```python
from build123d import *

# Parameters (mm, degrees)
BODY_MOVE_COPY1_START         = -65
BODY_MOVE_COPY1_OUTLINE_W     = 5.1
BODY_MOVE_COPY1_OUTLINE_H     = 30.1
BODY_MOVE_COPY1_OUTLINE_R     = 2.6
BODY_MOVE_COPY1_OUTLINE_R_2   = 3.1
BODY_MOVE_COPY1_OUTLINE_R_3   = 1.55
BODY_MOVE_COPY1_OUTLINE_W_2   = 30.5
BODY_MOVE_COPY1_OUTLINE_H_2   = 14.5
BODY_MOVE_COPY1_DEPTH         = 5
BODY_MOVE_COPY1_START_2       = -5
BODY_MOVE_COPY1_2_OUTLINE_W   = 10
BODY_MOVE_COPY1_2_OUTLINE_H   = 5.2
BODY_MOVE_COPY1_2_OUTLINE_R   = 1.6
BODY_MOVE_COPY1_2_OUTLINE_W_2 = 5.1
BODY_MOVE_COPY1_2_OUTLINE_H_2 = 30.1
BODY_MOVE_COPY1_2_DEPTH       = 5
SKETCH26_W                    = 10
SKETCH26_H                    = 5.2
BOSS_EXTRUDE2_DEPTH           = 5
SKETCH28_W                    = 5.1
SKETCH28_H                    = 30.1
CUT_EXTRUDE1_DEPTH            = 349.066085679


# Read off the part's stored shape, not the designer's step: Body-Move/Copy1
with BuildPart() as part:
    # Body-Move/Copy1 outline → Body-Move/Copy1 (new body)
    with BuildSketch(Plane.XY.offset(BODY_MOVE_COPY1_START)):
        Polygon((24.9, -310), (24.9, -305), (100.2, -305), (100.2, -310), (150, -310), (150, -5), (10.65, -5), (10.65, 0), (-10.65, 0), (-10.65, -5), (-150, -5), (-150, -310), (-100.2, -310), (-100.2, -305), (-24.9, -305), (-24.9, -310), align=None)
        with Locations((-143.45, -280)):
            Rectangle(BODY_MOVE_COPY1_OUTLINE_W, BODY_MOVE_COPY1_OUTLINE_H, mode=Mode.SUBTRACT)
        with Locations((-90, -157.5)):
            Circle(BODY_MOVE_COPY1_OUTLINE_R, mode=Mode.SUBTRACT)
        with Locations((-60, -157.5)):
            Circle(BODY_MOVE_COPY1_OUTLINE_R, mode=Mode.SUBTRACT)
        with Locations((143.45, -280)):
            Rectangle(BODY_MOVE_COPY1_OUTLINE_W, BODY_MOVE_COPY1_OUTLINE_H, mode=Mode.SUBTRACT)
        with Locations((65, -157.5)):
            Circle(BODY_MOVE_COPY1_OUTLINE_R_2, mode=Mode.SUBTRACT)
        with Locations((85, -157.5)):
            Circle(BODY_MOVE_COPY1_OUTLINE_R_2, mode=Mode.SUBTRACT)
        with Locations((-90, -137.5)):
            Circle(BODY_MOVE_COPY1_OUTLINE_R_3, mode=Mode.SUBTRACT)
        with Locations((-60, -137.5)):
            Circle(BODY_MOVE_COPY1_OUTLINE_R_3, mode=Mode.SUBTRACT)
        with Locations((-75, -100.25)):
            Rectangle(BODY_MOVE_COPY1_OUTLINE_W_2, BODY_MOVE_COPY1_OUTLINE_H_2, mode=Mode.SUBTRACT)
        with Locations((-143.45, -30)):
            Rectangle(BODY_MOVE_COPY1_OUTLINE_W, BODY_MOVE_COPY1_OUTLINE_H, mode=Mode.SUBTRACT)
        with Locations((143.45, -30)):
            Rectangle(BODY_MOVE_COPY1_OUTLINE_W, BODY_MOVE_COPY1_OUTLINE_H, mode=Mode.SUBTRACT)
    extrude(amount=BODY_MOVE_COPY1_DEPTH)


with BuildPart() as body_2:
    # Body-Move_Copy1 2 outline → Body-Move_Copy1 2 (new body)
    with BuildSketch(Plane(origin=(0, 0, 0), x_dir=(1, 0, 0), z_dir=(0, 1, 0)).offset(BODY_MOVE_COPY1_START_2)):
        with BuildLine():
            ThreePointArc((-95, -65), (-93.535533906, -61.464466094), (-90, -60))
            Line((-90, -60), (90, -60))
            ThreePointArc((90, -60), (93.535533906, -61.464466094), (95, -65))
            Line((95, -65), (95, -70))
            ThreePointArc((95, -70), (96.464466094, -73.535533906), (100, -75))
            Line((100, -75), (115, -75))
            ThreePointArc((115, -75), (118.535533906, -73.535533906), (120, -70))
            Line((120, -70), (120, -60))
            Line((120, -60), (145.606601718, -34.393398282))
            ThreePointArc((145.606601718, -34.393398282), (148.858192988, -29.52704805), (150, -23.786796564))
            Line((150, -23.786796564), (150, 65))
            Line((150, 65), (10.75, 65))
            Line((10.75, 65), (10.75, 60))
            Line((10.75, 60), (-10.75, 60))
            Line((-10.75, 60), (-10.75, 65))
            Line((-10.75, 65), (-150, 65))
            Line((-150, 65), (-150, -23.786796564))
            ThreePointArc((-150, -23.786796564), (-148.858192988, -29.52704805), (-145.606601718, -34.393398282))
            Line((-145.606601718, -34.393398282), (-120, -60))
            Line((-120, -60), (-120, -70))
            ThreePointArc((-120, -70), (-118.535533906, -73.535533906), (-115, -75))
            Line((-115, -75), (-100, -75))
            ThreePointArc((-100, -75), (-96.464466094, -73.535533906), (-95, -70))
            Line((-95, -70), (-95, -65))
        make_face()
        with Locations((-107.5, -67.5)):
            Rectangle(BODY_MOVE_COPY1_2_OUTLINE_W, BODY_MOVE_COPY1_2_OUTLINE_H, mode=Mode.SUBTRACT)
        with Locations((-110, -52.5)):
            Circle(BODY_MOVE_COPY1_2_OUTLINE_R, mode=Mode.SUBTRACT)
        with Locations((-5, -52.5)):
            Circle(BODY_MOVE_COPY1_2_OUTLINE_R, mode=Mode.SUBTRACT)
        with Locations((5, -52.5)):
            Circle(BODY_MOVE_COPY1_2_OUTLINE_R, mode=Mode.SUBTRACT)
        with Locations((107.5, -67.5)):
            Rectangle(BODY_MOVE_COPY1_2_OUTLINE_W, BODY_MOVE_COPY1_2_OUTLINE_H, mode=Mode.SUBTRACT)
        with Locations((110, -52.5)):
            Circle(BODY_MOVE_COPY1_2_OUTLINE_R, mode=Mode.SUBTRACT)
        with Locations((-143.45, 35)):
            Rectangle(BODY_MOVE_COPY1_2_OUTLINE_W_2, BODY_MOVE_COPY1_2_OUTLINE_H_2, mode=Mode.SUBTRACT)
        with Locations((-110, 52.5)):
            Circle(BODY_MOVE_COPY1_2_OUTLINE_R, mode=Mode.SUBTRACT)
        with Locations((-5, 52.5)):
            Circle(BODY_MOVE_COPY1_2_OUTLINE_R, mode=Mode.SUBTRACT)
        with BuildLine():
            Line((131.606601718, -30.178932188), (115.267766953, -46.517766953))
            ThreePointArc((115.267766953, -46.517766953), (114.456708581, -47.059698831), (113.5, -47.25))
            Line((113.5, -47.25), (107.75, -47.25))
            ThreePointArc((107.75, -47.25), (105.982233047, -47.982233047), (105.25, -49.75))
            Line((105.25, -49.75), (105.25, -53.5))
            ThreePointArc((105.25, -53.5), (104.517766953, -55.267766953), (102.75, -56))
            Line((102.75, -56), (13.25, -56))
            ThreePointArc((13.25, -56), (11.482233047, -55.267766953), (10.75, -53.5))
            Line((10.75, -53.5), (10.75, -49.75))
            ThreePointArc((10.75, -49.75), (10.017766953, -47.982233047), (8.25, -47.25))
            Line((8.25, -47.25), (-8.25, -47.25))
            ThreePointArc((-8.25, -47.25), (-10.017766953, -47.982233047), (-10.75, -49.75))
            Line((-10.75, -49.75), (-10.75, -53.5))
            ThreePointArc((-10.75, -53.5), (-11.482233047, -55.267766953), (-13.25, -56))
            Line((-13.25, -56), (-102.75, -56))
            ThreePointArc((-102.75, -56), (-104.517766953, -55.267766953), (-105.25, -53.5))
            Line((-105.25, -53.5), (-105.25, -49.75))
            ThreePointArc((-105.25, -49.75), (-105.982233047, -47.982233047), (-107.75, -47.25))
            Line((-107.75, -47.25), (-113.5, -47.25))
            ThreePointArc((-113.5, -47.25), (-115.267766953, -46.517766953), (-116, -44.75))
            Line((-116, -44.75), (-116, 44.75))
            ThreePointArc((-116, 44.75), (-115.267766953, 46.517766953), (-113.5, 47.25))
            Line((-113.5, 47.25), (-107.75, 47.25))
            ThreePointArc((-107.75, 47.25), (-105.982233047, 47.982233047), (-105.25, 49.75))
            Line((-105.25, 49.75), (-105.25, 53.5))
            ThreePointArc((-105.25, 53.5), (-104.517766953, 55.267766953), (-102.75, 56))
            Line((-102.75, 56), (-13.25, 56))
            ThreePointArc((-13.25, 56), (-11.482233047, 55.267766953), (-10.75, 53.5))
            Line((-10.75, 53.5), (-10.75, 49.75))
            ThreePointArc((-10.75, 49.75), (-10.017766953, 47.982233047), (-8.25, 47.25))
            Line((-8.25, 47.25), (8.25, 47.25))
            ThreePointArc((8.25, 47.25), (10.017766953, 47.982233047), (10.75, 49.75))
            Line((10.75, 49.75), (10.75, 53.5))
            ThreePointArc((10.75, 53.5), (11.482233047, 55.267766953), (13.25, 56))
            Line((13.25, 56), (102.75, 56))
            ThreePointArc((102.75, 56), (104.517766953, 55.267766953), (105.25, 53.5))
            Line((105.25, 53.5), (105.25, 49.75))
            ThreePointArc((105.25, 49.75), (105.982233047, 47.982233047), (107.75, 47.25))
            Line((107.75, 47.25), (113.5, 47.25))
            ThreePointArc((113.5, 47.25), (115.267766953, 47.982233047), (116, 49.75))
            Line((116, 49.75), (116, 53.5))
            ThreePointArc((116, 53.5), (116.732233047, 55.267766953), (118.5, 56))
            Line((118.5, 56), (133.5, 56))
            ThreePointArc((133.5, 56), (135.267766953, 55.267766953), (136, 53.5))
            Line((136, 53.5), (136, -19.57233047))
            ThreePointArc((136, -19.57233047), (134.858192988, -25.312581956), (131.606601718, -30.178932188))
        make_face(mode=Mode.SUBTRACT)
        with Locations((5, 52.5)):
            Circle(BODY_MOVE_COPY1_2_OUTLINE_R, mode=Mode.SUBTRACT)
        with Locations((143.45, 35)):
            Rectangle(BODY_MOVE_COPY1_2_OUTLINE_W_2, BODY_MOVE_COPY1_2_OUTLINE_H_2, mode=Mode.SUBTRACT)
        with Locations((110, 52.5)):
            Circle(BODY_MOVE_COPY1_2_OUTLINE_R, mode=Mode.SUBTRACT)
    extrude(amount=BODY_MOVE_COPY1_2_DEPTH)


with BuildPart() as body_3:
    # Sketch26 → Boss-Extrude2 (new body)
    with BuildSketch(Plane.XZ.offset(310)):
        with BuildLine():
            Line((-90, 60), (90, 60))
            ThreePointArc((90, 60), (93.535533906, 61.464466094), (95, 65))
            Line((95, 65), (95, 70))
            ThreePointArc((95, 70), (96.464466094, 73.535533906), (100, 75))
            Line((100, 75), (115, 75))
            ThreePointArc((115, 75), (118.535533906, 73.535533906), (120, 70))
            Line((120, 70), (120, 60))
            Line((120, 60), (145.606601718, 34.393398282))
            ThreePointArc((145.606601718, 34.393398282), (148.858192988, 29.52704805), (150, 23.786796564))
            Line((150, 23.786796564), (150, -60))
            Line((150, -60), (100.1, -60))
            Line((100.1, -60), (100.1, -65))
            Line((100.1, -65), (25, -65))
            Line((25, -65), (25, -60))
            Line((25, -60), (-25, -60))
            Line((-25, -60), (-25, -65))
            Line((-25, -65), (-100.1, -65))
            Line((-100.1, -65), (-100.1, -60))
            Line((-100.1, -60), (-150, -60))
            Line((-150, -60), (-150, 23.786796564))
            ThreePointArc((-150, 23.786796564), (-148.858192988, 29.52704805), (-145.606601718, 34.393398282))
            Line((-145.606601718, 34.393398282), (-120, 60))
            Line((-120, 60), (-120, 70))
            ThreePointArc((-120, 70), (-118.535533906, 73.535533906), (-115, 75))
            Line((-115, 75), (-100, 75))
            ThreePointArc((-100, 75), (-96.464466094, 73.535533906), (-95, 70))
            Line((-95, 70), (-95, 65))
            ThreePointArc((-95, 65), (-93.535533906, 61.464466094), (-90, 60))
        make_face()
        with Locations((107.5, 67.5)):
            Rectangle(SKETCH26_W, SKETCH26_H, mode=Mode.SUBTRACT)
        with Locations((-107.5, 67.5)):
            Rectangle(SKETCH26_W, SKETCH26_H, mode=Mode.SUBTRACT)
    extrude(amount=-BOSS_EXTRUDE2_DEPTH)

    # Sketch28 → Cut-Extrude1 (cut, through all)
    with BuildSketch(Plane(origin=(0, -305, 0), x_dir=(1, 0, 0), z_dir=(0, 1, 0))):
        with Locations((143.45, 35)):
            Rectangle(SKETCH28_W, SKETCH28_H)
        with Locations((-143.45, 35)):
            Rectangle(SKETCH28_W, SKETCH28_H)
    extrude(amount=-CUT_EXTRUDE1_DEPTH, mode=Mode.SUBTRACT)


solid = body_3.part
```
Check sheet for the modelled part. Datum: model origin and axes. Units: mm. A direction names the side the tool comes from. Round coordinates to 2 decimals unless told otherwise and drop trailing zeros. Order: outer loops, then holes, each group sorted by start corner. A loop starts at its lowest first (then second) coordinate and runs counter-clockwise, first axis right, second up. Notation, with made-up numbers: (-15, -10) -> (5, -10) arc R25 cw to (5, 14) -> close; hole circle Ø4 at (76.5, 11). An arc over 180 degrees is marked (long way). Use CSV: the item, a comma, the result in double quotes.
(1) Depth check by flat-ended pin: pin 1 (1.5 mm diameter, centred on x = -99.5, y = -306, fed in from +Z); pin 2 (2.5 mm diameter, centred on x = 108, y = -308.5, fed in from -Z); pin 3 (2.5 mm diameter, centred on y = -308.5, z = 67, fed in from +X); pin 4 (2.5 mm diameter, centred on x = 142.5, y = -307.5, fed in from +Z). Enter the tip coordinate at first touch or a pass-through.
Worked out:
pin 1,"z = 75"
pin 2,"z = -60"
pin 3,"x = 120"
pin 4,"z = 38.75"
(2) Cross-section at A-A (z = -31). Record the boundary of the cut face in (x, y), and give its area (3 significant figures).
Worked out:
outline,"(-150, -310) -> (-146, -310) -> (-146, -305) -> (-150, -305) -> close; (-140.9, -310) -> (140.9, -310) -> (140.9, -305) -> (-140.9, -305) -> close; (146, -310) -> (150, -310) -> (150, -305) -> (146, -305) -> close"
area,"1,450 mm²"
(3) Cross-section at C-C (y = -307.05). Count the separate pieces of the cut face and the enclosed holes in it, and give its area (3 significant figures).
Worked out:
separate pieces,"1"
enclosed holes,"4"
area,"36,200 mm²"
(4) Material ranges on line 1 along X through (y, z) = (-308.6, -46); line 2 along Z through (x, y) = (-103.5, -309.45); line 3 along X through (y, z) = (-305.95, 24), recorded low to high. Write a range as from..to.
Worked out:
line 1,"-150..-146, -140.9..140.9, 146..150"
line 2,"-60..64.9, 70.1..75"
line 3,"-150..150"
(5) Draft check along Z on faces 1 (the face through (93, -308, 61)), 2 (the face through (150, -308, -18)), 3 (the face through (107, -308, 64.9)). Enter one of: pulls with the +Z half, pulls with the -Z half, needs draft (parallel to the pull), parting line crosses it, or undercut.
Worked out:
face 1,"pulls with the +Z half"
face 2,"needs draft"
face 3,"undercut"
(6) Cross-section at B-B (x = 105.5). Record the boundary of the cut face in (y, z).
Worked out:
outline,"(-310, -60) -> (-305, -60) -> (-305, 64.9) -> (-310, 64.9) -> close; (-310, 70.1) -> (-305, 70.1) -> (-305, 75) -> (-310, 75) -> close"
(7) Cross-section at D-D (x = -28). Record the boundary of the cut face in (y, z).
Worked out:
outline,"(-310, -65) -> (-305, -65) -> (-305, 60) -> (-310, 60) -> close"
(8) Tool access check on faces 4 (the face through (-108, -308, 64.9)), 5 (the face through (-100.1, -308, -63)), 6 (the face through (-120, -308, 65)), 7 (the face through (25, -308, -63)), 8 (the face through (95, -308, 67)). Record the directions out of +Z, -Z, +X, -X, +Y, -Y that give a thin tool (end or side, any length) a straight path to the whole face; none if there is none.
Worked out:
face 4,"+Y, -Y"
face 5,"-Z, -X, +Y, -Y"
face 6,"+Z, -X, +Y, -Y"
face 7,"-Z, +Y, -Y"
face 8,"+Z, +Y, -Y"
